Geometry check sheet. Reference: the model listing, model coordinates, mm. Face numbers are marked on the shaded views. A direction names the side the tool comes from. Round coordinates to 2 decimals unless told otherwise and drop trailing zeros. Write each loop counter-clockwise with the first axis right and the second up, starting at its lowest first coordinate (ties: lowest second). Pieces come first, ordered by that corner, then holes.
Item 1: Access from +Z, -Z, +X, -X, +Y, -Y to the whole of each face (thin tool, end or side, straight path). Record for the marked faces 1 and 2.
Item 2: Depth check by flat-ended pin: P1, Ø2, axis at y = 42, z = -12.5, coming from the -X side; P2, Ø5, axis at x = 13, z = 0, coming from the +Y side; P3, Ø1, axis at y = 46.5, z = -8.5, coming from the +X side. Enter the tip coordinate at first touch or a pass-through.
Item 3: Cross-section at A-A (x = 0). Enter the section's corners in (y, z), then the cut area to 3 significant figures.
Item 4: Cross-section at B-B (z = 13). Enter the section's corners in (x, y), then the cut area to 3 significant figures.
Item 5: Cross-section at D-D (x = -6.5). Enter the section's corners in (y, z), then the cut area to 3 significant figures.
Item 6: Cross-section at C-C (y = 40). Enter the section's corners in (x, z).
Item 7: Scan lines: probe 1 along X at (y, z) = (73.5, 0); probe 2 along Y at (x, z) = (-10.5, -15.5). Record each from-to range of solid material in increasing order.
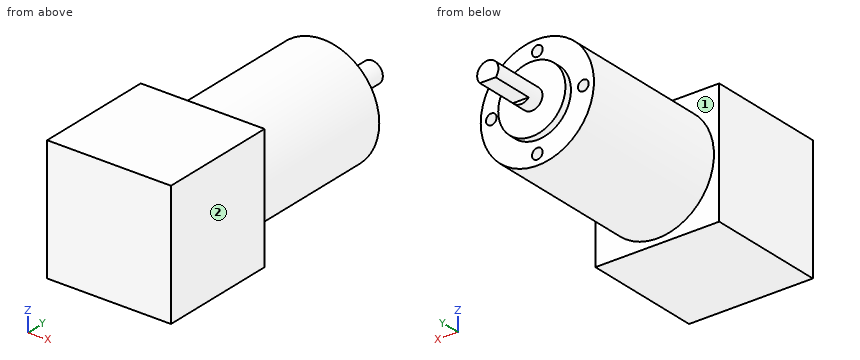
from build123d import *

# Parameters (mm, degrees)
SKETCH1_W           = 35
SKETCH1_H           = 35
BOSS_EXTRUDE1_DEPTH = 34
SKETCH2_R           = 16
BOSS_EXTRUDE2_DEPTH = 43.6
SKETCH3_R           = 9.5
BOSS_EXTRUDE3_DEPTH = 2
SKETCH4_R           = 3
BOSS_EXTRUDE4_DEPTH = 16
CUT_EXTRUDE1_DEPTH  = 12
SKETCH6_R           = 1.5
CUT_EXTRUDE2_DEPTH  = 7


with BuildPart() as part:
    # Sketch1 → Boss-Extrude1 (new body)
    with BuildSketch(Plane(origin=(0, 0, 0), x_dir=(1, 0, 0), z_dir=(0, 1, 0))):
        Rectangle(SKETCH1_W, SKETCH1_H)
    extrude(amount=BOSS_EXTRUDE1_DEPTH)

    # Sketch2 → Boss-Extrude2 (add)
    with BuildSketch(Plane(origin=(0, 34, 0), x_dir=(1, 0, 0), z_dir=(0, 1, 0))):
        Circle(SKETCH2_R)
    extrude(amount=BOSS_EXTRUDE2_DEPTH)

    # Sketch3 → Boss-Extrude3 (add)
    with BuildSketch(Plane(origin=(0, 77.6, 0), x_dir=(1, 0, 0), z_dir=(0, 1, 0))):
        Circle(SKETCH3_R)
    extrude(amount=BOSS_EXTRUDE3_DEPTH)

    # Sketch4 → Boss-Extrude4 (add)
    with BuildSketch(Plane(origin=(0, 79.6, 0), x_dir=(1, 0, 0), z_dir=(0, 1, 0))):
        Circle(SKETCH4_R)
    extrude(amount=BOSS_EXTRUDE4_DEPTH)

    # Sketch5 → Cut-Extrude1 (cut)
    with BuildSketch(Plane(origin=(0, 95.6, 0), x_dir=(1, 0, 0), z_dir=(0, 1, 0))):
        with BuildLine():
            Line((2.236067977, 2), (-2.236067977, 2))
            ThreePointArc((-2.236067977, 2), (0, 3), (2.236067977, 2))
        make_face()
    extrude(amount=-CUT_EXTRUDE1_DEPTH, mode=Mode.SUBTRACT)

    # Sketch6 → Cut-Extrude2 (cut)
    with BuildSketch(Plane(origin=(0, 77.6, 0), x_dir=(1, 0, 0), z_dir=(0, 1, 0))):
        with Locations((0, 13)):
            Circle(SKETCH6_R)
        with Locations((13, 0)):
            Circle(SKETCH6_R)
        with Locations((-13, 0)):
            Circle(SKETCH6_R)
        with Locations((0, -13)):
            Circle(SKETCH6_R)
    extrude(amount=-CUT_EXTRUDE2_DEPTH, mode=Mode.SUBTRACT)


solid = part.part
Resolved:
1. face 1: +Y
1. face 2: +Z, -Z, +X, +Y, -Y
2. P1: stops at x = -11.12
2. P2: stops at y = 77.6
2. P3: stops at x = 13.86
3. outline: (0, -17.5) - (34, -17.5) - (34, -16) - (77.6, -16) - (77.6, -14.5) - (70.6, -14.5) - (70.6, -11.5) - (77.6, -11.5) - (77.6, -9.5) - (79.6, -9.5) - (79.6, -3) - (83.6, -3) - (83.6, -2) - (95.6, -2) - (95.6, 3) - (79.6, 3) - (79.6, 9.5) - (77.6, 9.5) - (77.6, 11.5) - (70.6, 11.5) - (70.6, 14.5) - (77.6, 14.5) - (77.6, 16) - (34, 16) - (34, 17.5) - (0, 17.5) - close
3. area: 2,670 mm2
4. outline: (-17.5, 0) - (17.5, 0) - (17.5, 34) - (9.33, 34) - (9.33, 77.6) - (1.5, 77.6) - (1.5, 70.6) - (-1.5, 70.6) - (-1.5, 77.6) - (-9.33, 77.6) - (-9.33, 34) - (-17.5, 34) - close
4. area: 1,980 mm2
5. outline: (0, -17.5) - (34, -17.5) - (34, -14.62) - (77.6, -14.62) - (77.6, -6.93) - (79.6, -6.93) - (79.6, 6.93) - (77.6, 6.93) - (77.6, 14.62) - (34, 14.62) - (34, 17.5) - (0, 17.5) - close
5. area: 2,490 mm2
6. outline: circle Ø32 at (0, 0)
7. probe 1: x = -16 to -14.5, -11.5 to 11.5, 14.5 to 16
7. probe 2: y = 0 to 34
